```python
from build123d import *

# Parameters (mm, degrees)
F1_DEPTH = 50
F2_DEPTH = 50
F3_DEPTH = 18
F4_DEPTH = 18
F5_DEPTH = 31
F7_DEPTH = 205.001


with BuildPart() as f1:
    # F0 (on Top) → F1 (new body)
    with BuildSketch(Plane.XY):
        Polygon((0, 6), (0, 0), (205, 0), (205, 69), (195, 69), align=None)
    extrude(amount=-F1_DEPTH)

    # F0 (on Top) → F2 (join)
    with BuildSketch(Plane.XY):
        Polygon((0, 6), (0, 0), (205, 0), (205, 69), (195, 69), align=None)
    extrude(amount=F2_DEPTH)

    # F0 (on Top) → F3 (join)
    with BuildSketch(Plane.XY):
        Polygon((0, 16), (0, 6), (195, 69), (163.703159, 68.888713), align=None)
    extrude(amount=F3_DEPTH)

    # F3_face (on face) → F4 (join)
    with BuildSketch(Plane(origin=(89.903344, 39.900279, 0), x_dir=(1, 0, 0), z_dir=(0, 0, -1))):
        Polygon((105.096656, -29.099721), (-89.903344, 33.900279), (-89.903344, 23.900279), (73.799815, -28.988434), align=None)
    extrude(amount=F4_DEPTH)

    # F0 (on Top) → F5 (join, symmetric)
    with BuildSketch(Plane.XY):
        Polygon((0, 26), (0, 16), (163.703159, 68.888713), (133.095238, 69), align=None)
    extrude(amount=F5_DEPTH, both=True)

    # F6 (on Right) → F7 (cut, through all)
    with BuildSketch(Plane.YZ):
        with BuildLine():
            Line((0, 49.929991), (0, -50.243031))
            ThreePointArc((0, -50.243031), (4.000039, -0.15652), (0, 49.929991))
        make_face()
    extrude(amount=F7_DEPTH, mode=Mode.SUBTRACT)


solid = f1.part
```
Read the model definition and answer for the solid it produces. Units are mm, in the model's axes. A direction names the side the tool comes from. Give positions to 0.01 mm unless a question says otherwise; leave off trailing zeros. Write each loop counter-clockwise with the first axis right and the second up, starting at its lowest first coordinate (ties: lowest second). Pieces come first, ordered by that corner, then holes. Notation, with made-up numbers: M 45.25,19.25 L 79.25,19.25 A12 cw 79.25,39.25 Z; hole C 61.5,73 d8. An arc over 180 degrees is marked long. Put each result on its own line as item: value. Start each with the question number.
1. Which of the six approach directions +Z, -Z, +X, -X, +Y, -Y give full straight-line access (tool end or side, diameter ignored) to faces 1 (the flat face through (80.706, 42.074, 24.591)), 2 (the flat face through (75, 45, -31)), 3 (the flat face through (80.706, 42.074, -24.409))?
2. Consider line 1 along Z through (x, y) = (15, 13.5); line 2 along Y through (x, z) = (64.5, -28); line 3 along Y through (x, z) = (15.5, 19.5). Determine where each line is inside the solid, lowest interval first.
3. The part is cut by section B-B, the plane x = 182.5. Give the vertices of the cut face in (y, z), and give its area (3 significant figures).
4. The part is cut by section A-A, the plane z = 24. Give the vertices of the cut face in (x, y), and give its area (3 significant figures).
5. Each of these flat-tipped pins is pushed along its axis until it touches: pin 1 Ø4 at (x, z) = (129, 16.5) entering from +Y; pin 2 Ø1 at (x, z) = (108.5, 30.5) entering from +Y; pin 3 Ø19 at (x, y) = (117.5, 49) entering from -Z; pin 4 Ø2 at (x, z) = (181, -20.5) entering from +Y. Where does it stop, or does it pass through?
6. For a pull along Y with two mould halves and no side action, classify faces 4 (the cylindrical face through (101, 4, -1)), 5 (the flat face through (90, 40, 18)), 6 (the flat face through (0, 13, 1)) as released by +Y, released by -Y, zero draft, split by the parting line, or undercut.
7. The part is cut by section D-D, the plane z = -39. Give the vertices of the cut face in (x, y).
8. The part is cut by section C-C, the plane y = 64.5. Give the vertices of the cut face in (x, z), and give its area (3 significant figures).
Final values:
1. face 1: +Z
1. face 2: -Z, -X, +Y
1. face 3: -Z
2. line 1: z = -18 to 18
2. line 2: y = 2.77 to 26.84, 36.84 to 46.84
2. line 3: y = 3.39 to 11.01, 21.01 to 31.01
3. outline: M 0,49.93 A315.58 cw 0.04,-50 L 64.96,-50 L 64.96,-18 L 68.96,-18 L 68.96,18 L 64.96,18 L 64.96,50 L 0,50 Z
3. area: 6,370 mm²
4. outline: M 0,3.07 L 205,3.07 L 205,69 L 195,69 L 0,6 Z; M 0,16 L 163.7,68.89 L 133.1,69 L 0,26 Z
4. area: 8,860 mm²
5. pin 1: stops at y = 68.32
5. pin 2: stops at y = 61.22
5. pin 3: stops at z = -50
5. pin 4: stops at y = 64.8
6. face 4: released by -Y
6. face 5: undercut
6. face 6: zero draft
7. outline: M 0,1.6 L 205,1.6 L 205,69 L 195,69 L 0,6 Z
8. outline: M 119.17,-31 L 150.12,-31 L 150.12,-18 L 181.07,-18 L 181.07,-50 L 205,-50 L 205,50 L 181.07,50 L 181.07,18 L 150.12,18 L 150.12,31 L 119.17,31 Z
8. area: 5,430 mm²
